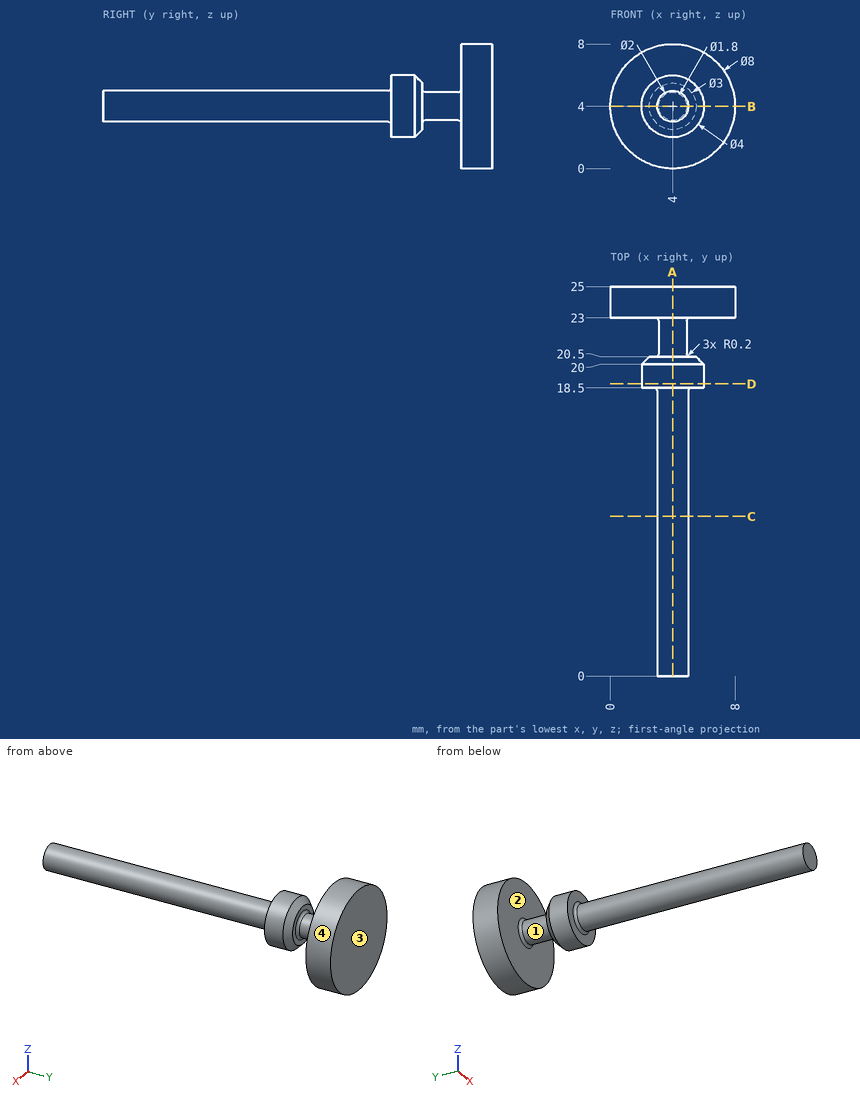
Verification items for this drawing (mm, ordinates from the low corner). Give positions to 0.01 mm unless a question says otherwise; leave off trailing zeros. Write each loop counter-clockwise with the first axis right and the second up, starting at its lowest first coordinate (ties: lowest second). Pieces come first, ordered by that corner, then holes. Notation, with made-up numbers: (27, 8.5) -> (32, 8.5) arc R21 ccw to (32, 20.5) -> close; hole circle Ø11 at (1, 61.5). An arc over 180 degrees is marked (long way). Use CSV: the item, a comma, the result in double quotes.
(1) Material ranges on L1, parallel to Y at x = 7.25, z = 6; L2, parallel to Y at x = 5.5, z = 5; L3, parallel to Z at x = 4.25, y = 15, recorded low to high.
Derived:
L1,"y = 23 to 25"
L2,"y = 18.5 to 20.2, 23 to 25"
L3,"z = 3.03 to 4.97"
(2) Go/stop test with flat-tipped pins: pin 1 (2 mm diameter, centred on x = 4.5, y = 17, fed in from -Z); pin 2 (3 mm diameter, centred on x = 3.5, y = 18, fed in from -Z); pin 3 (4 mm diameter, centred on x = 1, z = 2, fed in from -Y). Record where each tip stops, or that it passes through.
Derived:
pin 1,"stops at z = 3"
pin 2,"stops at z = 2"
pin 3,"stops at y = 18.5"
(3) Sectioned sample at D-D (y = 18.75). Record the cut outline in (x, z).
Derived:
outline,"circle Ø4 at (4, 4)"
(4) Release check for a two-part mould opening along Y. For the marked faces 1, 2, 3 and 4 record: +Y half, -Y half, draft (parallel to the pull), parting line (faces both ways), or undercut.
Derived:
face 1,"undercut"
face 2,"undercut"
face 3,"+Y half"
face 4,"draft"
(5) Sectioned sample at B-B (z = 4). Record the cut outline in (x, y), plus the area to 3 significant figures.
Derived:
outline,"(0, 23) -> (2.9, 23) arc R0.2 cw to (3.1, 22.8) -> (3.1, 20.7) arc R0.2 cw to (2.9, 20.5) -> (2.5, 20.5) -> (2, 20) -> (2, 18.5) -> (2.8, 18.5) arc R0.2 cw to (3, 18.3) -> (3, 0) -> (5, 0) -> (5, 18.3) arc R0.2 cw to (5.2, 18.5) -> (6, 18.5) -> (6, 20) -> (5.5, 20.5) -> (5.1, 20.5) arc R0.2 cw to (4.9, 20.7) -> (4.9, 22.8) arc R0.2 cw to (5.1, 23) -> (8, 23) -> (8, 25) -> (0, 25) -> close"
area,"65.3 mm^2"
(6) Sectioned sample at A-A (x = 4). Record the cut outline in (y, z).
Derived:
outline,"(0, 3) -> (18.3, 3) arc R0.2 cw to (18.5, 2.8) -> (18.5, 2) -> (20, 2) -> (20.5, 2.5) -> (20.5, 2.9) arc R0.2 cw to (20.7, 3.1) -> (22.8, 3.1) arc R0.2 cw to (23, 2.9) -> (23, 0) -> (25, 0) -> (25, 8) -> (23, 8) -> (23, 5.1) arc R0.2 cw to (22.8, 4.9) -> (20.7, 4.9) arc R0.2 cw to (20.5, 5.1) -> (20.5, 5.5) -> (20, 6) -> (18.5, 6) -> (18.5, 5.2) arc R0.2 cw to (18.3, 5) -> (0, 5) -> close"
(7) Sectioned sample at C-C (y = 10.25). Record the cut outline in (x, z), plus the area to 3 significant figures.
Derived:
outline,"circle Ø2 at (4, 4)"
area,"3.14 mm^2"
